Here's how the part is built. I have some questions about the finished solid (model axes, mm). Face numbers are marked on the shaded views. A direction names the side the tool comes from. Round coordinates to 2 decimals unless told otherwise and drop trailing zeros. Order: outer loops, then holes, each group sorted by start corner. A loop starts at its lowest first (then second) coordinate and runs counter-clockwise, first axis right, second up. Notation, with made-up numbers: (57.5, -16) - (114.5, -16) arc R11 cw to (114.5, -3) - close; hole circle Ø10 at (22, 63). An arc over 180 degrees is marked (long way). Answer as a JSON object with one key per item and string values.
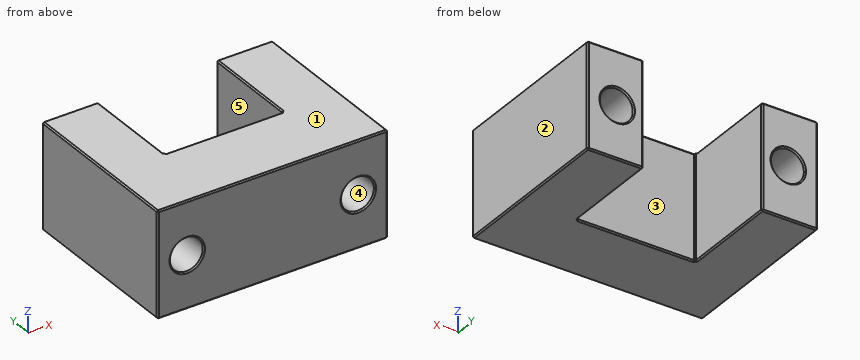
```python
from build123d import *

# Parameters (mm, degrees)
BOSS_EXTRUDE1_DEPTH = 8
SKETCH2_R           = 2.5
CUT_EXTRUDE1_DEPTH  = 33.345787979
CHAMFER1_SIZE       = 0.2


with BuildPart() as part:
    # Sketch1 → Boss-Extrude1 (new, symmetric)
    with BuildSketch(Plane.XY):
        Polygon((0, 0), (-17.5, 0), (-17.5, 26), (-9, 26), (-9, 11), (0, 11), align=None)
    boss_extrude1 = extrude(amount=BOSS_EXTRUDE1_DEPTH, both=True)

    # Mirror1: Boss-Extrude1 across plane
    add(boss_extrude1.mirror(Plane(origin=(0, 0, 0), x_dir=(0, 0, 1), z_dir=(1, 0, 0))))

    # Sketch2 → Cut-Extrude1 (cut, through all)
    with BuildSketch(Plane(origin=(0, 26, 0), x_dir=(1, 0, 0), z_dir=(0, 1, 0))):
        with Locations(Location((-13, 0, 0), (0, 0, 270))):
            Circle(SKETCH2_R)
        with Locations(Location((13, 0, 0), (0, 0, 270))):
            Circle(SKETCH2_R)
    extrude(amount=-CUT_EXTRUDE1_DEPTH, mode=Mode.SUBTRACT)

    # Chamfer1
    chamfer1_edges = [part.edges().sort_by_distance(p)[0] for p in [
        (-17.5, 0, 0),
        (-17.5, 26, 0),
        (-9, 26, 0),
        (-9, 11, 0),
        (-9, 18.5, 8),
        (-13.25, 26, 8),
        (17.5, 13, 8),
        (-17.5, 13, 8),
        (17.5, 0, 0),
        (13.25, 26, 8),
        (17.5, 26, 0),
        (9, 18.5, 8),
        (9, 26, 0),
        (9, 11, 0),
        (9, 18.5, -8),
        (13.25, 26, -8),
        (17.5, 13, -8),
        (0, 0, 8),
        (-13, 0, -2.5),
        (-13, 26, -2.5),
        (13, 0, -2.5),
        (13, 26, -2.5),
        (0, 0, -8),
        (-17.5, 13, -8),
        (-13.25, 26, -8),
        (-9, 18.5, -8),
        (0, 11, -8),
        (0, 11, 8),
    ]]
    chamfer(chamfer1_edges, length=CHAMFER1_SIZE)


solid = part.part
```
1. If I drill on L1, parallel to X at y = 16.75, z = 0; L2, parallel to X at y = 24.25, z = 4.75; L3, parallel to Y at x = 5, z = -4, over which ranges is the centre line in solid material (lowest first)? Write a range as [from, to].
Responses:
{"L1": "[-17.5, -15.5], [-10.5, -9], [9, 10.5], [15.5, 17.5]", "L2": "[-17.5, -9], [9, 17.5]", "L3": "[0, 11]"}
2. Imagine slicing it at B-B (x = -13). List the corners of the cut face in (y, z) for me, plus the area to 3 significant figures.
Responses:
{"outline": "(0, -7.8) - (0.2, -8) - (25.8, -8) - (26, -7.8) - (26, -2.7) - (25.8, -2.5) - (0.2, -2.5) - (0, -2.7) - close; (0, 2.7) - (0.2, 2.5) - (25.8, 2.5) - (26, 2.7) - (26, 7.8) - (25.8, 8) - (0.2, 8) - (0, 7.8) - close", "area": "286 mm2"}
3. Imagine slicing it at C-C (z = 0). Give the number of separate pieces and of enclosed holes in the cut face, plus the area to 3 significant figures.
Responses:
{"separate pieces": "3", "enclosed holes": "0", "area": "380 mm2"}
4. For the marked faces 4 and 5, which set-ups out of +Z, -Z, +X, -X, +Y, -Y let a thin tool reach every point of the face, with its end or its side?
Responses:
{"face 4": "+Y, -Y", "face 5": "+Z, -Z, +Y"}
5. Imagine slicing it at D-D (y = 8.25). List the corners of the cut face in (x, z) for me, plus the area to 3 significant figures.
Responses:
{"outline": "(-17.5, -7.8) - (-17.3, -8) - (17.3, -8) - (17.5, -7.8) - (17.5, 7.8) - (17.3, 8) - (-17.3, 8) - (-17.5, 7.8) - close; hole circle Ø5 at (-13, 0); hole circle Ø5 at (13, 0)", "area": "521 mm2"}
6. Thinking about a two-plate mould opening in X: for the marked faces 1, 2 and 3, which applies, pulls with the +X half, pulls with the -X half, needs draft (parallel to the pull), parting line crosses it, or undercut?
Responses:
{"face 1": "needs draft", "face 2": "pulls with the +X half", "face 3": "undercut"}
7. Imagine slicing it at A-A (y = 21). List the corners of the cut face in (x, z) for me, plus the area to 3 significant figures.
Responses:
{"outline": "(-17.5, -7.8) - (-17.3, -8) - (-9.2, -8) - (-9, -7.8) - (-9, 7.8) - (-9.2, 8) - (-17.3, 8) - (-17.5, 7.8) - close; (9, -7.8) - (9.2, -8) - (17.3, -8) - (17.5, -7.8) - (17.5, 7.8) - (17.3, 8) - (9.2, 8) - (9, 7.8) - close; hole circle Ø5 at (-13, 0); hole circle Ø5 at (13, 0)", "area": "233 mm2"}
8. For P1, Ø6, axis at x = 1, z = 5, coming from the +Y side, with a flat end and sliding along its axis, tell me the tip position at first contact or that it passes through.
Responses:
{"P1": "y = 11"}
